Can you work these out from the model? Positions are in its coordinate system, mm. Face numbers are marked on the shaded views. A direction names the side the tool comes from. Give positions to 0.01 mm unless a question says otherwise; leave off trailing zeros. Write each loop counter-clockwise with the first axis right and the second up, starting at its lowest first coordinate (ties: lowest second). Pieces come first, ordered by that corner, then holes. Notation, with made-up numbers: (48, 81) - (69, 81) arc R9 cw to (69, 97) - close; hole circle Ø4 at (24.25, -22.75). An arc over 180 degrees is marked (long way). Use a Markdown table: item, result. Add a question column.
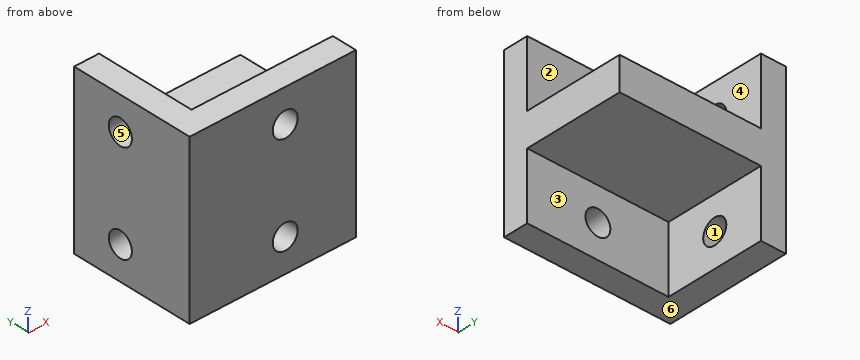
```python
from build123d import *

# Parameters (mm, degrees)
EXTRUDE_1_DEPTH     = 20
SKETCH_2_R          = 1.5
CUT_EXTRUDE_1_DEPTH = 29.861739379
SKETCH_3_R          = 1.5
CUT_EXTRUDE_2_DEPTH = 29.861739379
SKETCH_4_W          = 4
SKETCH_4_H          = 12
EXTRUDE_2_DEPTH     = 17


with BuildPart() as part:
    # 草图1 → 凸台-拉伸1 (new body)
    with BuildSketch(Plane.XY):
        Polygon((0, 0), (0, 12), (-3, 12), (-3, -3), (17, -3), (17, 0), align=None)
    extrude(amount=EXTRUDE_1_DEPTH)

    # 草图2 → 切除-拉伸1 (cut, through all)
    with BuildSketch(Plane(origin=(0, 0, 0), x_dir=(0, 0, -1), z_dir=(1, 0, 0))):
        with Locations(Location((-16, 6, 0), (0, 0, 90))):
            Circle(SKETCH_2_R)
        with Locations(Location((-4, 6, 0), (0, 0, 270))):
            Circle(SKETCH_2_R)
    extrude(amount=-CUT_EXTRUDE_1_DEPTH, mode=Mode.SUBTRACT)

    # 草图3 → 切除-拉伸2 (cut, through all)
    with BuildSketch(Plane(origin=(0, 0, 0), x_dir=(1, 0, 0), z_dir=(0, 1, 0))):
        with Locations(Location((8.5, -16, 0), (0, 0, 180))):
            Circle(SKETCH_3_R)
        with Locations((8.5, -4)):
            Circle(SKETCH_3_R)
    extrude(amount=-CUT_EXTRUDE_2_DEPTH, mode=Mode.SUBTRACT)

    # 草图4 → 凸台-拉伸2 (add)
    with BuildSketch(Plane(origin=(0, 0, 0), x_dir=(0, 0, -1), z_dir=(1, 0, 0))):
        with Locations((-10, 6)):
            Rectangle(SKETCH_4_W, SKETCH_4_H)
    extrude(amount=EXTRUDE_2_DEPTH)


solid = part.part
```
Q1. Suppose I cut it at B-B (y = 6). Please give me the cut outline in (x, z), and give its area (3 significant figures).
Q2. If we mould it in two halves opening along Z, with no side actions, what happens to the marked faces 4, 5 and 6? For each: released by +Z, released by -Z, zero draft, split by the parting line, or undercut.
Q3. I'm going to push flat-ended pins straight in: P1, Ø4, axis at x = 9, z = 4, coming from the +Y side; P2, Ø2.5, axis at x = 8.5, z = 16, coming from the +Y side; P3, Ø6.5, axis at y = 6, z = 16, coming from the +X side. Where does each tip first touch, or does it pass through?
Q4. Suppose I cut it at D-D (z = 13.75). Please give me the cut outline in (x, y).
Q5. Suppose I cut it at A-A (z = 16). Please give me the cut outline in (x, y), and give its area (3 significant figures).
Q6. If I drill on probe 1 along Z at (x, y) = (-1.75, 6); probe 2 along Y at (x, z) = (-1.35, 4); probe 3 along X at (y, z) = (-1.15, 4), over which ranges is the centre line in solid material (lowest first)? Write a range as [from, to].
Q7. On a 3-axis mill with a long thin cutter (end or side, diameter ignored), from which of +Z, -Z, +X, -X, +Y, -Y can I reach the whole of each face in a straight line? I mean the marked faces 1, 2 and 3. Say none if no direction works.
Q8. Suppose I cut it at C-C (x = 8.75). Please give me the cut outline in (y, z).
Derived:
| question | item | result |
|---|---|---|
| 1 | outline | (-3, 0) - (0, 0) - (0, 2.5) - (-3, 2.5) - close; (-3, 5.5) - (0, 5.5) - (0, 8) - (17, 8) - (17, 12) - (0, 12) - (0, 14.5) - (-3, 14.5) - close; (-3, 17.5) - (0, 17.5) - (0, 20) - (-3, 20) - close |
| 1 | area | 110 mm² |
| 2 | face 4 | zero draft |
| 2 | face 5 | undercut |
| 2 | face 6 | released by -Z |
| 3 | P1 | y = 0 |
| 3 | P2 | through |
| 3 | P3 | x = 0 |
| 4 | outline | (-3, -3) - (17, -3) - (17, 0) - (0, 0) - (0, 12) - (-3, 12) - close |
| 5 | outline | (-3, -3) - (7, -3) - (7, 0) - (0, 0) - (0, 4.5) - (-3, 4.5) - close; (-3, 7.5) - (0, 7.5) - (0, 12) - (-3, 12) - close; (10, -3) - (17, -3) - (17, 0) - (10, 0) - close |
| 5 | area | 78.0 mm² |
| 6 | probe 1 | [0, 2.5], [5.5, 14.5], [17.5, 20] |
| 6 | probe 2 | [-3, 4.5], [7.5, 12] |
| 6 | probe 3 | [-3, 7], [10, 17] |
| 7 | face 1 | +X, -X |
| 7 | face 2 | +Z, +X, +Y |
| 7 | face 3 | -Z, +X, +Y |
| 8 | outline | (-3, 0) - (0, 0) - (0, 2.52) - (-3, 2.52) - close; (-3, 5.48) - (0, 5.48) - (0, 8) - (12, 8) - (12, 12) - (0, 12) - (0, 14.52) - (-3, 14.52) - close; (-3, 17.48) - (0, 17.48) - (0, 20) - (-3, 20) - close |
